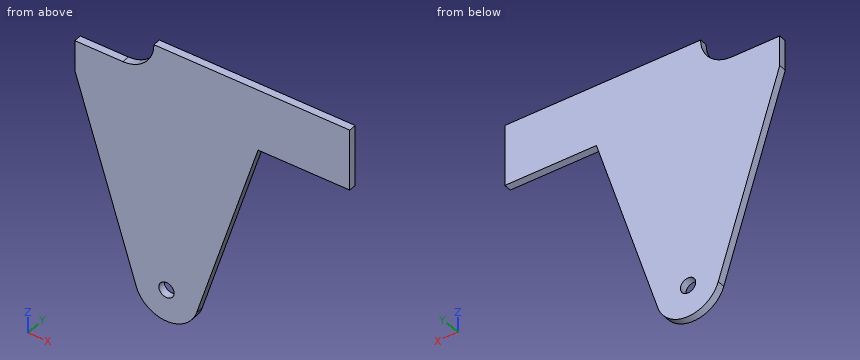
```python
from build123d import *

# Parameters (mm, degrees)
SKETCH1_R           = 6.35
BOSS_EXTRUDE1_DEPTH = 6.35


with BuildPart() as part:
    # Sketch1 → Boss-Extrude1 (new body)
    with BuildSketch(Plane(origin=(0, 0, 0), x_dir=(1, 0, 0), z_dir=(0, 1, 0))):
        with BuildLine():
            Line((76.2, -152.4), (25.106996492, 7.99757633))
            ThreePointArc((25.106996492, 7.99757633), (0, 26.35), (-25.106996492, 7.99757633))
            Line((-25.106996492, 7.99757633), (-76.2, -152.4))
            Line((-76.2, -152.4), (-76.2, -177.4))
            Line((-76.2, -177.4), (-36.2, -177.4))
            ThreePointArc((-36.2, -177.4), (-17.956645045, -184.956645045), (-10.4, -203.2))
            Line((-10.4, -203.2), (152.4, -203.2))
            Line((152.4, -203.2), (152.4, -152.4))
            Line((152.4, -152.4), (76.2, -152.4))
        make_face()
        Circle(SKETCH1_R, mode=Mode.SUBTRACT)
    extrude(amount=BOSS_EXTRUDE1_DEPTH)


solid = part.part
```
For this review, take the finished solid that the model builds, in its own axes (mm). Coordinates: 2 decimals unless noted, no trailing zeros. Write each loop counter-clockwise with the first axis right and the second up, starting at its lowest first coordinate (ties: lowest second). Pieces come first, ordered by that corner, then holes. Notation, with made-up numbers: (18.5, 86) - (64.5, 86) arc R18 ccw to (64.5, 110) - close; hole circle Ø8 at (89.25, -11). An arc over 180 degrees is marked (long way). Answer in a Markdown table with one row per item. Add a question column.
Q1. For probe 1 along Z at (x, y) = (0, 4); probe 2 along Z at (x, y) = (81, 1); probe 3 along Z at (x, y) = (8, 3), list the stretches that pass through material, from the lowest coordinate up.
Q2. We need section B-B, the plane x = 0. State the section outline as (y, z) points.
Q3. For P1, Ø1.9, axis at x = -64.5, y = 2.5, coming from the +Z side; P2, Ø1.5, axis at y = 4, z = 139.5, coming from the +X side; P3, Ø2, axis at y = 5.5, z = 101.5, coming from the -X side, all flat-tipped, find the tip position at first contact; note any pin that passes through.
Q4. We need section C-C, the plane z = 0. State the section outline as (x, y) points.
Q5. We need section A-A, the plane y = 1.5. State the section outline as (x, z) points.
Q6. We need section D-D, the plane x = 108. State the section outline as (y, z) points, and give its area (3 significant figures).
Answer list:
| question | item | result |
|---|---|---|
| 1 | probe 1 | z = -26.35 to -6.35, 6.35 to 203.2 |
| 1 | probe 2 | z = 152.4 to 203.2 |
| 1 | probe 3 | z = -25.11 to 203.2 |
| 2 | outline | (0, -26.35) - (6.35, -26.35) - (6.35, -6.35) - (0, -6.35) - close; (0, 6.35) - (6.35, 6.35) - (6.35, 203.2) - (0, 203.2) - close |
| 3 | P1 | stops at z = 177.4 |
| 3 | P2 | stops at x = 72.33 |
| 3 | P3 | stops at x = -60.3 |
| 4 | outline | (-27.65, 0) - (-6.35, 0) - (-6.35, 6.35) - (-27.65, 6.35) - close; (6.35, 0) - (27.65, 0) - (27.65, 6.35) - (6.35, 6.35) - close |
| 5 | outline | (-76.2, 152.4) - (-25.11, -8) arc R26.35 ccw to (25.11, -8) - (76.2, 152.4) - (152.4, 152.4) - (152.4, 203.2) - (-10.4, 203.2) arc R25.8 cw to (-36.2, 177.4) - (-76.2, 177.4) - close; hole circle Ø12.7 at (0, 0) |
| 6 | outline | (0, 152.4) - (6.35, 152.4) - (6.35, 203.2) - (0, 203.2) - close |
| 6 | area | 323 mm2 |
